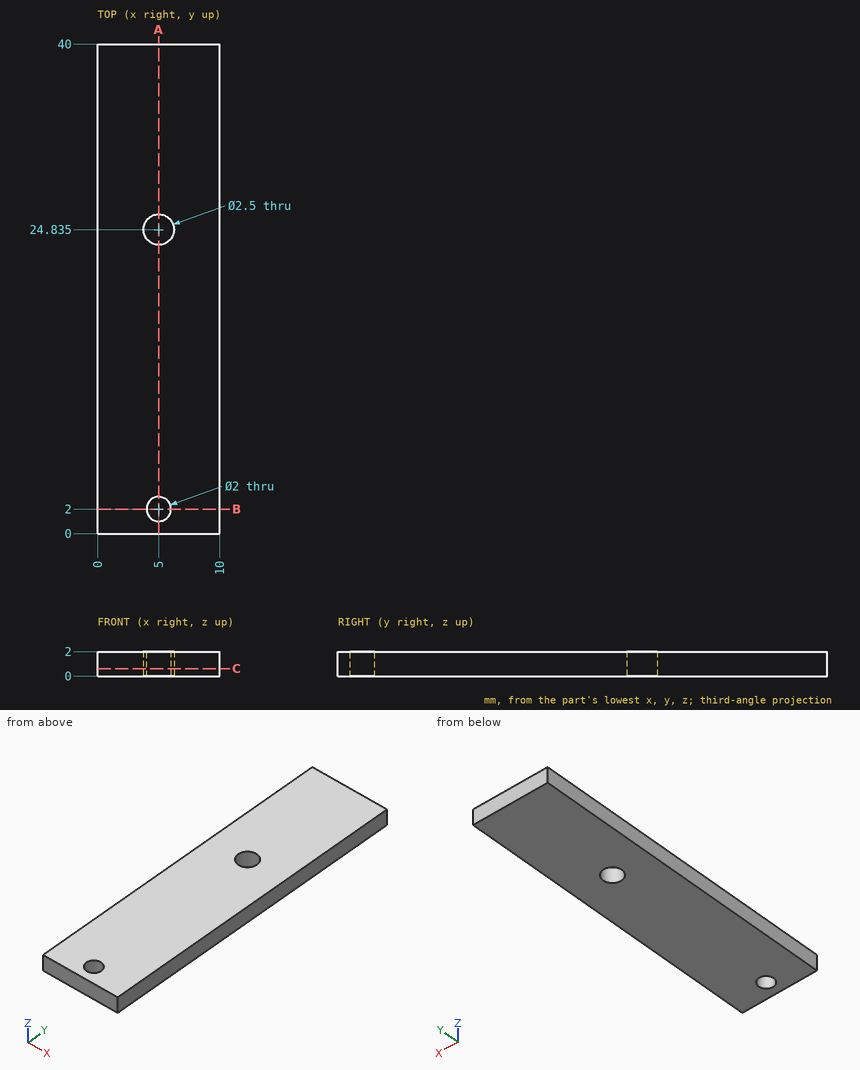
The figure shows three views and two pictorial views of one solid part (mm, origin at its lowest corner). Answer the questions. Give positions to 0.01 mm unless a question says otherwise; leave off trailing zeros. Write each loop counter-clockwise with the first axis right and the second up, starting at its lowest first coordinate (ties: lowest second). Pieces come first, ordered by that corner, then holes.
Q1. Given pin 1 (4 mm diameter, centred on x = 5, y = 24.84, fed in from -Z); pin 2 (1.8 mm diameter, centred on x = 5, y = 2, fed in from -Z), each flat-ended and moving along its own axis, determine where each tip first touches the part or whether it passes through.
Answer:
pin 1: stops at z = 0
pin 2: passes through
Q2. Straight lines are drawn through the part: L1, parallel to Y at x = 5, z = 0.85 (3 decimals); L2, parallel to Y at x = 4.25, z = 1.3 (1 decimal); L3, parallel to X at y = 25, z = 1.1. For each, find the intervals that lie inside material, in ascending order.
Answer:
L1: y = 0 to 1, 3 to 23.585, 26.085 to 40
L2: y = 0 to 1.3, 2.7 to 23.8, 25.8 to 40
L3: x = 0 to 3.76, 6.24 to 10
Q3. The part is cut by section A-A on x = 5. Give the vertices of the cut face in (y, z) (3 decimals), and give its area (3 significant figures).
Answer:
outline: (0, 0) - (1, 0) - (1, 2) - (0, 2) - close; (3, 0) - (23.585, 0) - (23.585, 2) - (3, 2) - close; (26.085, 0) - (40, 0) - (40, 2) - (26.085, 2) - close
area: 71.0 mm2
Q4. The part is cut by section C-C on z = 0.6. Give the vertices of the cut face in (x, y) (3 decimals), and give its area (3 significant figures).
Answer:
outline: (0, 0) - (10, 0) - (10, 40) - (0, 40) - close; hole circle Ø2.5 at (5, 24.835); hole circle Ø2 at (5, 2)
area: 392 mm2
Q5. The part is cut by section B-B on y = 2. Give the vertices of the cut face in (x, z), and give its area (3 significant figures).
Answer:
outline: (0, 0) - (4, 0) - (4, 2) - (0, 2) - close; (6, 0) - (10, 0) - (10, 2) - (6, 2) - close
area: 16.0 mm2
